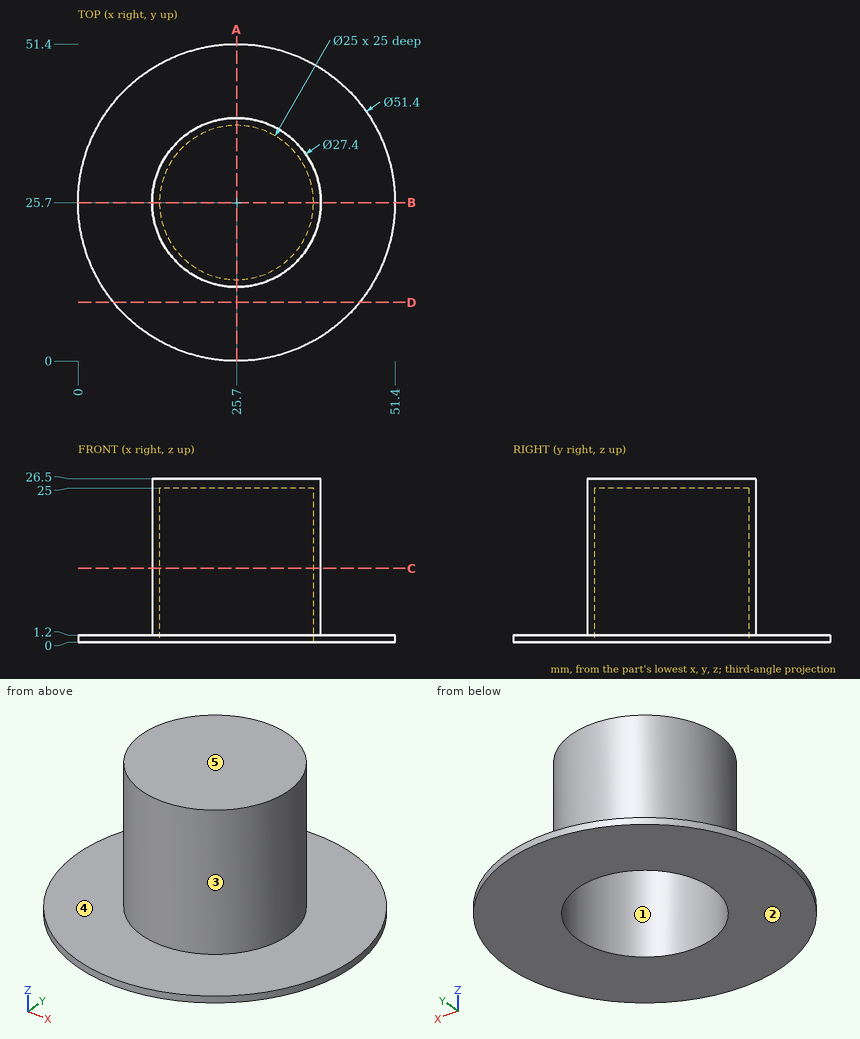
Job drawing, mm, ordinate dimensions from the low corner. One solid piece. A direction names the side the tool comes from. Coordinates: 2 decimals unless noted, no trailing zeros. Loops run counter-clockwise (first coordinate to the right, second up) from the corner with the lowest first, then second, coordinate; pieces in that order, holes last. Notation, with made-up numbers: (-33, -4.5) - (-16, -4.5) arc R24 ccw to (-16, 10.5) - close; hole circle Ø10 at (58.5, 30.25). An arc over 180 degrees is marked (long way). Answer as a JSON object with one key per item and string values. Group by question number.
(1) Two-plate mould, pull along X, no slides. Class the marked faces 1, 2 and 3: released by +X, released by -X, zero draft, split by the parting line, or undercut.
(2) Flat gauge pins, fed straight in: pin 1 (2 mm diameter, centred on x = 8.5, y = 35.5, fed in from +Z); pin 2 (6 mm diameter, centred on y = 39, z = 11, fed in from +X); pin 3 (10 mm diameter, centred on y = 5.5, z = 3, fed in from -X). Where does each tip first touch, or does it go through?
(3) Cut at C-C (z = 12). Give the cut face in (x, y).
(4) Probe line 1 along Y through (x, z) = (25.7, 15.5); line 2 along Z through (x, y) = (5.5, 31). List the from-to ranges inside material, lowest first.
(5) Tool access for the marked faces 4 and 5: list every direction of +Z, -Z, +X, -X, +Y, -Y with a clear straight run to the whole face (end or side of a thin tool).
(6) Cut at A-A (x = 25.7). Give the cut face in (y, z), then the cut area to 3 significant figures.
(7) Cut at D-D (y = 9.5). Give the cut face in (x, z), then the cut area to 3 significant figures.
Geometry says:
{
 "1": {"face 1": "undercut", "face 2": "zero draft", "face 3": "split by the parting line"},
 "2": {"pin 1": "stops at z = 1.2", "pin 2": "stops at x = 34.73", "pin 3": "stops at x = 5.23"},
 "3": {"outline": "circle Ø27.4 at (25.7, 25.7); hole circle Ø25 at (25.7, 25.7)"},
 "4": {"line 1": "y = 12 to 13.2, 38.2 to 39.4", "line 2": "z = 0 to 1.2"},
 "5": {"face 4": "+Z", "face 5": "+Z, +X, -X, +Y, -Y"},
 "6": {"outline": "(0, 0) - (13.2, 0) - (13.2, 25) - (38.2, 25) - (38.2, 0) - (51.4, 0) - (51.4, 1.2) - (39.4, 1.2) - (39.4, 26.5) - (12, 26.5) - (12, 1.2) - (0, 1.2) - close", "area": "130 mm^2"},
 "7": {"outline": "(5.75, 0) - (45.65, 0) - (45.65, 1.2) - (5.75, 1.2) - close", "area": "47.9 mm^2"}
}
